from build123d import *

# Parameters (mm, degrees)
SKETCH1_W           = 16
SKETCH1_H           = 14
BOSS_EXTRUDE1_DEPTH = 3


with BuildPart() as part:
    # Sketch1 → Boss-Extrude1 (new body)
    with BuildSketch(Plane(origin=(0, 0, 0), x_dir=(1, 0, 0), z_dir=(0, 1, 0))):
        with Locations((-34.802547771, 15.318471338)):
            Rectangle(SKETCH1_W, SKETCH1_H)
        with BuildLine():
            Line((-39.747765047, 14.717010334), (-33.675750706, 14.717010334))
            add(Edge.make_bspline(
                [(-39.747765047, 14.717010334), (-39.561120933, 17.701061711), (-33.79747245, 17.731175732), (-33.675750706, 14.717010334)],
                knots=[0, 0, 0, 0, 1, 1, 1, 1], degree=3))
        make_face(mode=Mode.SUBTRACT)
        with BuildLine():
            Line((-38.965889228, 14.351025908), (-34.357812591, 14.351025908))
            ThreePointArc((-34.357812591, 14.351025908), (-33.875378575, 13.868591892), (-34.357812591, 13.386157876))
            Line((-34.357812591, 13.386157876), (-38.965889228, 13.386157876))
            ThreePointArc((-38.965889228, 13.386157876), (-39.448323244, 13.868591892), (-38.965889228, 14.351025908))
        make_face(mode=Mode.SUBTRACT)
        with BuildLine():
            Line((-39.533825085, 12.024167234), (-33.838965327, 12.024167234))
            Line((-33.838965327, 12.024167234), (-34.443549741, 11.294520332))
            ThreePointArc((-34.443549741, 11.294520332), (-34.788137861, 11.027556057), (-35.213561017, 10.932550609))
            Line((-35.213561017, 10.932550609), (-38.507427743, 10.932550609))
            ThreePointArc((-38.507427743, 10.932550609), (-39.157744536, 11.172887481), (-39.495471122, 11.778374472))
            Line((-39.495471122, 11.778374472), (-39.533825085, 12.024167234))
        make_face(mode=Mode.SUBTRACT)
        with BuildLine():
            Line((-38.965889228, 12.521103778), (-38.965889228, 12.254933286))
            Line((-38.965889228, 12.254933286), (-34.357812591, 12.254933286))
            Line((-34.357812591, 12.254933286), (-34.357812591, 12.521103778))
            ThreePointArc((-34.357812591, 12.521103778), (-34.840246607, 12.916411942), (-35.322680624, 12.521103778))
            ThreePointArc((-35.322680624, 12.521103778), (-35.721936361, 12.920359515), (-36.121192098, 12.521103778))
            ThreePointArc((-36.121192098, 12.521103778), (-36.487176524, 12.887088204), (-36.85316095, 12.521103778))
            ThreePointArc((-36.85316095, 12.521103778), (-37.227463204, 12.895406032), (-37.601765458, 12.521103778))
            ThreePointArc((-37.601765458, 12.521103778), (-37.951114229, 12.870452548), (-38.300462999, 12.521103778))
            ThreePointArc((-38.300462999, 12.521103778), (-38.633176113, 12.853816892), (-38.965889228, 12.521103778))
        make_face(mode=Mode.SUBTRACT)
        with BuildLine():
            Line((-34.945417172, 10.384522547), (-34.635673461, 8.779972828))
            Line((-34.635673461, 8.779972828), (-31.865915017, 8.779972828))
            Line((-31.865915017, 8.779972828), (-30.414179557, 16.573500036))
            Line((-30.414179557, 16.573500036), (-33.675750706, 16.573500036))
            add(Edge.make_bspline(
                [(-33.675750706, 16.573500036), (-32.735887192, 14.661705952), (-32.525301104, 11.881425098), (-34.357812591, 10.384522547)],
                knots=[0, 0, 0, 0, 1, 1, 1, 1], degree=3))
            Line((-34.357812591, 10.384522547), (-34.945417172, 10.384522547))
        make_face(mode=Mode.SUBTRACT)
        Polygon((-34.357812591, 16.993739248), (-30.165856386, 16.993739248), (-30.165856386, 17.815115891), (-35.322680624, 17.815115891), align=None, mode=Mode.SUBTRACT)
        with BuildLine():
            Line((-33.473024699, 18.033096236), (-32.744268505, 18.033096236))
            Line((-32.744268505, 18.033096236), (-32.419866706, 19.916311952))
            Line((-32.419866706, 19.916311952), (-30.414179557, 20.317449381))
            Line((-30.414179557, 20.317449381), (-30.414179557, 20.9478082))
            Line((-30.414179557, 20.9478082), (-33.250794239, 20.380485263))
            Line((-33.250794239, 20.380485263), (-33.655154301, 18.033096236))
            ThreePointArc((-33.655154301, 18.033096236), (-33.5640895, 18.025310185), (-33.473024699, 18.033096236))
        make_face(mode=Mode.SUBTRACT)
    extrude(amount=BOSS_EXTRUDE1_DEPTH)


solid = part.part
Model file for the job. Use its own axes, mm. A direction names the side the tool comes from. Give positions to 0.01 mm unless a question says otherwise; leave off trailing zeros. Order: outer loops, then holes, each group sorted by start corner. A loop starts at its lowest first (then second) coordinate and runs counter-clockwise, first axis right, second up. Notation, with made-up numbers: M 59,-25.75 L 72,-25.75 A29 cw 72,8.25 Z; hole C -7.5,12 d8. An arc over 180 degrees is marked long. Put each result on its own line as item: value. Start each with the question number.
(1) Band-saw the part on B-B on y = 1.65. Count the separate pieces of the cut face and the enclosed holes in it, then the cut area to 3 significant figures.
(2) Pin check, flat tip, straight feed: pin 1 Ø3 at (x, z) = (-38.5, -11) entering from +Y. Stop position of the tip, or through.
(3) Pull direction X, two halves, no side cores. Call faces 3 (the face through (-34.847, 1.479, -17.41)), 4 (the face through (-35, 1, -22.318)), 5 (the face through (-42.803, 1, -15)): released by +X, released by -X, zero draft, split by the parting line, or undercut.
(4) Drill centre lines: L1, parallel to Z at x = -36.5, y = 1.3; L2, parallel to Z at x = -38.75, y = 0.5; L3, parallel to X at y = 0.7, z = -16. Where is each one in solid material? Low to high. Write a range as [from, to].
(5) Band-saw the part on A-A on x = -31. Give the cut face in (y, z).
(6) Tool access for faces 1 (the face through (-35, 0, -17)), 2 (the face through (-39.15, 1.479, -11.166)): list every direction of +Z, -Z, +X, -X, +Y, -Y with a clear straight run to the whole face (end or side of a thin tool).
Results below:
1. separate pieces: 1
1. enclosed holes: 7
1. area: 174 mm2
2. pin 1: stops at y = 3
3. face 3: undercut
3. face 4: zero draft
3. face 5: released by -X
4. L1: z = [-22.32, -16.96], [-14.72, -14.35], [-13.39, -12.89], [-12.25, -12.02], [-10.93, -8.32]
4. L2: z = [-22.32, -16.39], [-14.72, -14.35], [-13.39, -12.83], [-12.25, -12.02], [-10.96, -8.32]
4. L3: x = [-42.8, -39.21], [-34.18, -33.43], [-30.52, -26.8]
5. outline: M 0,-22.32 L 3,-22.32 L 3,-20.83 L 0,-20.83 Z; M 0,-20.2 L 3,-20.2 L 3,-17.82 L 0,-17.82 Z; M 0,-16.99 L 3,-16.99 L 3,-16.57 L 0,-16.57 Z; M 0,-13.43 L 3,-13.43 L 3,-8.32 L 0,-8.32 Z
6. face 1: +Z, -Z, +X, -X, -Y
6. face 2: +Y, -Y
